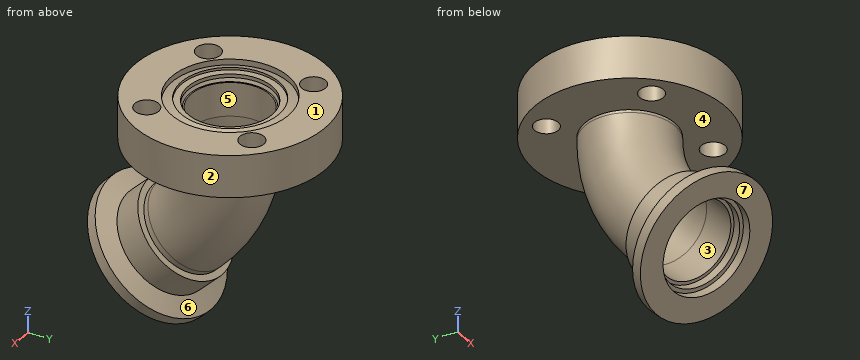
from build123d import *

# Parameters (mm, degrees)
SKETCH3_R          = 3.3655
CUT_EXTRUDE2_DEPTH = 40.896285426
CIRPATTERN1_COUNT  = 4
SKETCH6_R          = 12.7
SKETCH6_R_2        = 11.049


with BuildPart() as part:
    # Sketch1 → Revolve1 (revolve)
    with BuildSketch(Plane(origin=(0, 0, 0), x_dir=(0, 0, -1), z_dir=(1, 0, 0)), mode=Mode.PRIVATE) as revolve1_sk:
        Polygon((0, 26.924), (0, 16.51), (1.624198303, 16.51), (0.635, 13.7922), (1.3208, 13.7922), (1.3208, 11.9126), (2.3368, 11.9126), (3.722613851, 11.1125), (11.9126, 11.1125), (11.9126, 26.924), align=None)
    revolve(revolve1_sk.sketch.rotate(Axis((0, 0, 0), (0, 0, -1)), 90), axis=Axis((0, 0, 0), (0, 0, -1)))

    # Sketch3 → Cut-Extrude2 (cut, through all)
    with BuildSketch(Plane.XY):
        with Locations((14.593532367, 14.5923)):
            Circle(SKETCH3_R)
    cut_extrude2 = extrude(amount=-CUT_EXTRUDE2_DEPTH, mode=Mode.SUBTRACT)

    # CirPattern1: Cut-Extrude2 ×4 about axis
    cirpattern1_axis = Axis((0, 0, 0), (0, 0, 1))
    for i in range(1, CIRPATTERN1_COUNT):
        add(cut_extrude2.rotate(cirpattern1_axis, i * 360 / CIRPATTERN1_COUNT), mode=Mode.SUBTRACT)

    # Sweep2: sweep along a path in Sketch5
    with BuildLine(Plane(origin=(0, 0, 0), x_dir=(0, 0, -1), z_dir=(1, 0, 0))) as sweep2_path:
        Line((3.175, 0), (12.7, 0))
        ThreePointArc((12.7, 0), (27.280238773, -2.900189811), (39.640768363, -11.159231637))
        Line((39.640768363, -11.159231637), (46.375960454, -17.894423728))
    # Sketch6 → Sweep2 (sweep)
    with BuildSketch(Plane.XY.offset(-3.175)):
        Circle(SKETCH6_R)
        Circle(SKETCH6_R_2, mode=Mode.SUBTRACT)
    sweep(path=sweep2_path.line)

    # Sketch7 → Revolve2 (revolve)
    with BuildSketch(Plane(origin=(0, 0, 0), x_dir=(0, 0, -1), z_dir=(1, 0, 0)), mode=Mode.PRIVATE) as revolve2_sk:
        Polygon((56.431890618, -10.999543718), (57.224109848, -10.207324488), (59.020161072, -12.003375712), (63.88745989, -7.136076895), (61.732198421, -4.980815425), (56.833518782, -7.809069434), (51.043736945, -2.019287597), (49.247685721, -3.815338821), align=None)
    revolve(revolve2_sk.sketch.rotate(Axis((0, -17.894423728, -46.375960454), (0, -0.7071067811865475, -0.7071067811865476)), 180), axis=Axis((0, -17.894423728, -46.375960454), (0, -0.7071067811865475, -0.7071067811865476)))


solid = part.part
CAD build for the part. Positions are in the model's coordinates, mm. Face numbers are marked on the shaded views. A direction names the side the tool comes from. Coordinates: 2 decimals unless noted, no trailing zeros. Write each loop counter-clockwise with the first axis right and the second up, starting at its lowest first coordinate (ties: lowest second). Pieces come first, ordered by that corner, then holes. Notation, with made-up numbers: M 49,76.25 L 65,76.25 A12 ccw 65,95.25 Z; hole C -31.5,67.25 d3. An arc over 180 degrees is marked long. Answer as a JSON object with one key per item and string values. Group by question number.
1) Mould opens along Z. For the marked faces 1, 2, 3 and 4 say: +Z half, -Z half, draft (parallel to the pull), parting line (faces both ways), or undercut.
2) Wall check: line 1 (Y direction, x = 0, z = -10.5); line 2 (Z direction, x = -23, y = -12.5); line 3 (Y direction, x = -7, z = -34). Give the ranges that are in metal, low to high. Write a range as from..to.
3) Tool access for the marked faces 5, 6 and 7: list every direction of +Z, -Z, +X, -X, +Y, -Y with a clear straight run to the whole face (end or side of a thin tool).
4) Saw through at A-A (z = -4.5). Write the cut outline in (x, y), plus the area to 3 significant figures.
5) Pin check, flat tips, straight feed: pin 1 Ø9 at (x, y) = (-14.59, 14.59) entering from -Z; pin 2 Ø7.5 at (x, y) = (-14.59, -14.59) entering from -Z; pin 3 Ø11 at (x, y) = (14.59, -14.59) entering from -Z. Stop position of each tip, or through.
Values follow:
{
 "1": {"face 1": "+Z half", "face 2": "draft", "face 3": "undercut", "face 4": "undercut"},
 "2": {"line 1": "y = -26.92..-11.05, 11.05..26.92", "line 2": "z = -11.91..0", "line 3": "y = -23.52..-17.61, 3.4..5.69"},
 "3": {"face 5": "+Z", "face 6": "none", "face 7": "-Z, +X, -X, -Y"},
 "4": {"outline": "C 0,0 d53.85; hole C -14.59,-14.59 d6.73; hole C -14.59,14.59 d6.73; hole C 0,0 d22.1; hole C 14.59,-14.59 d6.73; hole C 14.59,14.59 d6.73", "area": "1,750 mm2"},
 "5": {"pin 1": "stops at z = -11.91", "pin 2": "stops at z = -60.07", "pin 3": "stops at z = -61.17"}
}
